Geometry check sheet. Reference: the model listing, model coordinates, mm. Give positions to 0.01 mm unless a question says otherwise; leave off trailing zeros. Order: outer loops, then holes, each group sorted by start corner. A loop starts at its lowest first (then second) coordinate and runs counter-clockwise, first axis right, second up.
Autodesk Inventor part; units mm, degrees
ref_plane "Work Plane1" through (-18.9656, 0, 0) normal (0, -0.8660254, -0.5) x (1, 0, 0)
ref_plane "YZ Plane" through (0, 0, 0) normal (1, 0, 0) x (0, 1, 0)
ref_plane "XZ Plane" through (0, 0, 0) normal (0, 1, 0) x (-1, 0, 0)
sketch "Эскиз1" plane through (0, 0, 0) normal (1, 0, 0) x (0, 1, 0)
  line L0 (-10.3923, 0) -> (-5.1962, 9)
  line L1 (-5.1962, 9) -> (5.1962, 9)
  line L2 (5.1962, 9) -> (10.3923, 0)
  line L3 (10.3923, 0) -> (5.1962, -9)
  line L4 (5.1962, -9) -> (-5.1962, -9)
  line L5 (-5.1962, -9) -> (-10.3923, 0)
  point P0 (0, 0)
  point P1 (0, 0)
  dimension "d0" = 20.7846
extrude "Базовый элемент" add sketch "Эскиз1" along normal blind 10.8
sketch "Эскиз2" plane through (0, 0, 0) normal (0, 0, 1) x (1, 0, 0)
  line L0 (0, 5.1962) -> (0, 10.3923)
  line L1 (0, 10.3923) -> (10.8, 10.3923)
  line L2 (10.8, 5.1962) -> (10.8, 10.3923)
  line L3 (-2.16, 0) -> (12.96, 0)
  line L4 (1.1993, 10.3923) -> (0, 8.315)
  line L5 (9.6007, 10.3923) -> (10.8, 8.315)
  dimension "d3" = 30
  dimension "d4" = 30
  dimension "d5" = 16.63
  dimension "d6" = 16.63
revolve "Фаска1" cut sketch "Эскиз2" angle 360 about axis through (-10, 0, 0) along (1, 0, 0)
sketch "Эскиз3" plane through (10.8, 0, 0) normal (1, 0, 0) x (0, 0, -1)
  arc A0 (-0.625, -1.0825) -> (0.625, -1.0825) centre (0, 0) ccw
hole "Резьба" at (10.8, 0, 0) direction (-1, 0, 0) diameter 10.647 end through all
chamfer "Фаска2" distance 0.6766 angle 30 1 edges at (10.8, 0, 5.3235) measured on face at (10.8, 7.2244, -0.8772)
chamfer "Фаска3" distance 0.6766 angle 30 1 edges at (0, 0, 5.3235) measured on face at (0, 7.2244, -0.8772)
ref_plane "Work Plane1" through (-18.9656, 0, 0) normal (0, -0.8660254, -0.5) x (1, 0, 0)
equation "\"d0\" = 1.1547 * SW"
equation "\"d1\" = KOH"
equation "\"d3\" = ANG1"
equation "\"d4\" = ANG2"
equation "\"d5\" = SW0"
equation "\"d6\" = SW01"
equation "\"d8\" = -0.5 * GD1 + 0.5 * NND"
equation "\"d40\" = -0.5 * GD1 + 0.5 * NND"
equation "\"d10\" = -0.5 * GD1 + 0.5 * NND"
equation "\"d41\" = -0.5 * GD1 + 0.5 * NND"
equation "\"ANG1\" = 30deg"
equation "\"ANG2\" = 30deg"
equation "\"NND\" = 12"
equation "\"KOH\" = 10.8"
equation "\"SW\" = 18"
equation "\"SW0\" = 16.63"
equation "\"SW01\" = SW0"
equation "\"GUL\" = 0.541266 * PTC"
equation "\"LADI\" = 16.63"
equation "\"TOA\" = 30deg"
equation "\"FAWI\" = 30deg"
equation "\"PTC\" = 1.25"
equation "\"THREADDIA\" = 12"
equation "\"E0\" = 1.155 * SW"
equation "\"GAL\" = 0.541266 * PTC"
properties part number "Копия гайки M12x1,25-6H ГОСТ 5915-70" material "Сталь, мягкая"
Q1. Cross-section at C-C, the plane x = 10. Record the boundary of the cut face in (y, z).
Q2. Thickness scan on L1, parallel to Z at x = 5.25, y = 0; L2, parallel to Y at x = 4.5, z = -3.75; L3, parallel to Z at x = 9.5, y = 2. Record the ranges inside material, lowest first.
Q3. Release check for a two-part mould opening along Y. For faces 1 (the face through (5, 0, 9)), 2 (the face through (5.33, 7.76, 4.56)), 3 (the face through (5.33, 2.039, -4.918)) record: pulls with the +Y half, pulls with the -Y half, needs draft (parallel to the pull), parting line crosses it, or undercut.
Q4. Cross-section at B-B, the plane x = 3.25. Record the boundary of the cut face in (y, z), and give its area (3 significant figures).
Q5. Gauge pin test, flat ends, axial feed: P1, Ø1.5, axis at x = 8.5, z = 7, coming from the +Y side; P2, Ø5, axis at x = 2.5, z = -4.5, coming from the -Y side; P3, Ø3, axis at x = 4, z = 3, coming from the -Y side. Record the tip position at first contact, or that the pin passes through.
Q6. Cross-section at A-A, the plane y = 0. Record the boundary of the cut face in (x, z) (1 decimal).
Answers follow:
1. outline: (-9.6, -1.37) - (-5.98, -7.63) arc R9.7 ccw to (-3.62, -9) - (3.62, -9) arc R9.7 ccw to (5.98, -7.63) - (9.6, -1.37) arc R9.7 ccw to (9.6, 1.37) - (5.98, 7.63) arc R9.7 ccw to (3.62, 9) - (-3.62, 9) arc R9.7 ccw to (-5.98, 7.63) - (-9.6, 1.37) arc R9.7 ccw to start; hole circle Ø10.65 at (0, 0)
2. L1: z = -9 to -5.32, 5.32 to 9
2. L2: y = -8.23 to -3.78, 3.78 to 8.23
2. L3: z = -9 to -4.93, 4.93 to 9
3. face 1: needs draft
3. face 2: pulls with the +Y half
3. face 3: undercut
4. outline: (-10.39, 0) - (-5.2, -9) - (5.2, -9) - (10.39, 0) - (5.2, 9) - (-5.2, 9) - close; hole circle Ø10.65 at (0, 0)
4. area: 192 mm2
5. P1: stops at y = 6.78
5. P2: stops at y = -9.24
5. P3: stops at y = -9.53
6. outline: (0, -8.3) - (0.4, -9) - (10.4, -9) - (10.8, -8.3) - (10.8, -6) - (10.4, -5.3) - (0.4, -5.3) - (0, -6) - close; (0, 6) - (0.4, 5.3) - (10.4, 5.3) - (10.8, 6) - (10.8, 8.3) - (10.4, 9) - (0.4, 9) - (0, 8.3) - close
